```python
from build123d import *

# Parameters (mm, degrees)
F0_R     = 19.05
F0_R_2   = 6.35
F1_DEPTH = 38.1
F2_DEPTH = 12.7
F3_DEPTH = 6.35


with BuildPart() as f1:
    # F0 (on Top) → F1 (new body)
    with BuildSketch(Plane.XY):
        with BuildLine():
            ThreePointArc((-837.6395976841, 421.923872186), (-821.3424535269, 430.1577150999), (-814.7795976841, 447.1965530885))
            ThreePointArc((-814.7795976841, 447.1965530885), (-821.3424535269, 464.235391077), (-837.6395976841, 472.469233991))
            ThreePointArc((-837.6395976841, 472.469233991), (-865.5795976841, 447.1965530885), (-837.6395976841, 421.923872186))
        make_face()
        with Locations((-840.1795976841, 447.1965530885)):
            Circle(F0_R, mode=Mode.SUBTRACT)
        with BuildLine():
            ThreePointArc((-837.6395976841, 472.469233991), (-821.3424535269, 464.235391077), (-814.7795976841, 447.1965530885))
            ThreePointArc((-814.7795976841, 447.1965530885), (-821.3424535269, 430.1577150999), (-837.6395976841, 421.923872186))
            Line((-837.6395976841, 421.923872186), (-711.9095976841, 434.5602126372))
            ThreePointArc((-711.9095976841, 434.5602126372), (-725.8795976841, 447.1965530885), (-711.9095976841, 459.8328935397))
            Line((-711.9095976841, 459.8328935397), (-837.6395976841, 472.469233991))
        make_face()
        with BuildLine():
            ThreePointArc((-802.0795976841, 440.6483835481), (-808.6277672246, 447.1965530885), (-802.0795976841, 453.7447226289))
            Line((-802.0795976841, 453.7447226289), (-751.2795976841, 453.7447226289))
            ThreePointArc((-751.2795976841, 453.7447226289), (-744.7314281437, 447.1965530885), (-751.2795976841, 440.6483835481))
            Line((-751.2795976841, 440.6483835481), (-802.0795976841, 440.6483835481))
        make_face(mode=Mode.SUBTRACT)
        with BuildLine():
            ThreePointArc((-700.4795976841, 447.1965530885), (-703.7610256055, 455.7159720828), (-711.9095976841, 459.8328935397))
            ThreePointArc((-711.9095976841, 459.8328935397), (-725.8795976841, 447.1965530885), (-711.9095976841, 434.5602126372))
            ThreePointArc((-711.9095976841, 434.5602126372), (-703.7610256055, 438.6771340942), (-700.4795976841, 447.1965530885))
        make_face()
        with Locations((-713.1795976841, 447.1965530885)):
            Circle(F0_R_2, mode=Mode.SUBTRACT)
    extrude(amount=F1_DEPTH)

    # F0 (on Top) → F2 (cut)
    with BuildSketch(Plane.XY):
        with BuildLine():
            ThreePointArc((-837.6395976841, 472.469233991), (-821.3424535269, 464.235391077), (-814.7795976841, 447.1965530885))
            ThreePointArc((-814.7795976841, 447.1965530885), (-821.3424535269, 430.1577150999), (-837.6395976841, 421.923872186))
            Line((-837.6395976841, 421.923872186), (-711.9095976841, 434.5602126372))
            ThreePointArc((-711.9095976841, 434.5602126372), (-725.8795976841, 447.1965530885), (-711.9095976841, 459.8328935397))
            Line((-711.9095976841, 459.8328935397), (-837.6395976841, 472.469233991))
        make_face()
        with BuildLine():
            ThreePointArc((-802.0795976841, 440.6483835481), (-808.6277672246, 447.1965530885), (-802.0795976841, 453.7447226289))
            Line((-802.0795976841, 453.7447226289), (-751.2795976841, 453.7447226289))
            ThreePointArc((-751.2795976841, 453.7447226289), (-744.7314281437, 447.1965530885), (-751.2795976841, 440.6483835481))
            Line((-751.2795976841, 440.6483835481), (-802.0795976841, 440.6483835481))
        make_face(mode=Mode.SUBTRACT)
    extrude(amount=F2_DEPTH, mode=Mode.SUBTRACT)

    # F3 (cut): a face of the model
    f3_faces = [f1.faces().sort_by_distance(p)[0] for p in [
        (-714.4136766597, 459.4754838588, 0),
    ]]
    extrude(f3_faces, amount=-F3_DEPTH, mode=Mode.SUBTRACT)


solid = f1.part
```
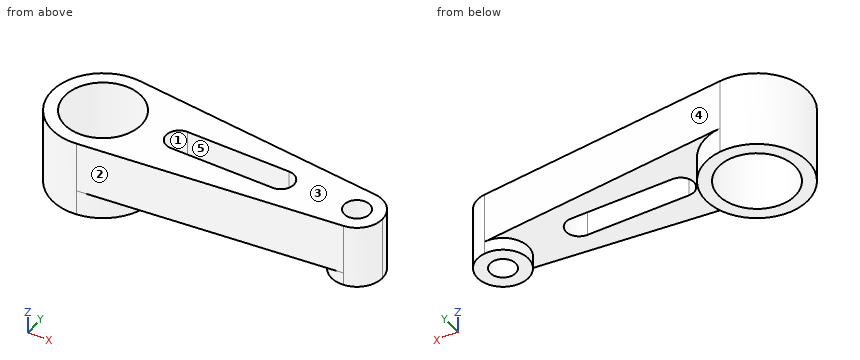
Verification items for the finished model (mm, model axes). Face numbers are marked on the shaded views. A direction names the side the tool comes from. Coordinates: 2 decimals unless noted, no trailing zeros. Write each loop counter-clockwise with the first axis right and the second up, starting at its lowest first coordinate (ties: lowest second). Pieces come first, ordered by that corner, then holes. Notation, with made-up numbers: (-1, 63) - (14, 63) arc R12 cw to (14, 81) - close; hole circle Ø4 at (21.25, 58.5). An arc over 180 degrees is marked (long way). Write item = value, one per line.
Q1. Mould release check, pull along Y, two halves, no side actions. Record for the marked faces 3, 4 and 5: released by +Y, released by -Y, zero draft, split by the parting line, or undercut.
Answer:
face_3 = zero draft
face_4 = released by +Y
face_5 = undercut
Q2. Access from +Z, -Z, +X, -X, +Y, -Y to the whole of each face (thin tool, end or side, straight path). Record for the marked faces 1 and 2.
Answer:
face_1 = +Z, -Z
face_2 = +Z, -Z, +X, -Y
Q3. Cross-section at B-B (x = -766). Enter the section's corners in (y, z), plus the area to 3 significant figures.
Answer:
outline = (429.12, 12.7) - (440.65, 12.7) - (440.65, 38.1) - (429.12, 38.1) - close; (453.74, 12.7) - (465.27, 12.7) - (465.27, 38.1) - (453.74, 38.1) - close
area = 585 mm²
Q4. Cross-section at C-C (y = 458). Enter the section's corners in (x, z), plus the area to 3 significant figures.
Answer:
outline = (-863.17, 0) - (-855.87, 0) - (-855.87, 38.1) - (-863.17, 38.1) - close; (-824.49, 0) - (-817.19, 0) - (-817.19, 12.7) - (-719.86, 12.7) - (-719.86, 6.35) - (-706.5, 6.35) - (-706.5, 38.1) - (-824.49, 38.1) - close
area = 3,450 mm²
Q5. Material ranges on L1, parallel to X at y = 445, z = 21.5; L2, parallel to X at y = 442, z = 15.5; L3, parallel to Z at x = -788.5, y = 435, recorded low to high. Write a range as from..to.
Answer:
L1 = -865.48..-859.1, -821.26..-808.25, -745.11..-719.14, -707.22..-700.67
L2 = -865.04..-858.51, -821.85..-806.06, -747.3..-716.83, -709.53..-701.59
L3 = 12.7..38.1
Q6. Cross-section at A-A (z = 8). Enter the section's corners in (x, y), plus the area to 3 significant figures.
Answer:
outline = circle Ø50.8 at (-840.18, 447.2); circle Ø25.4 at (-713.18, 447.2); hole circle Ø38.1 at (-840.18, 447.2); hole circle Ø12.7 at (-713.18, 447.2)
area = 1,270 mm²
Q7. Cross-section at D-D (z = 35). Enter the section's corners in (x, y), plus the area to 3 significant figures.
Answer:
outline = (-837.64, 421.92) - (-711.91, 434.56) arc R12.7 ccw to (-711.91, 459.83) - (-837.64, 472.47) arc R25.4 ccw (long way) to start; hole circle Ø38.1 at (-840.18, 447.2); hole (-802.08, 440.65) - (-751.28, 440.65) arc R6.55 ccw to (-751.28, 453.74) - (-802.08, 453.74) arc R6.55 ccw to start; hole circle Ø12.7 at (-713.18, 447.2)
area = 4,060 mm²
Q8. Go/stop test with flat-tipped pins: pin 1 Ø12 at (x, y) = (-768.5, 431.5) entering from -Z; pin 2 Ø3 at (x, z) = (-753.5, 19) entering from +Y; pin 3 Ø20.5 at (x, y) = (-712.5, 449.5) entering from -Z. Record where each tip stops, or that it passes through.
Answer:
pin_1 = 12.7
pin_2 = 464.16
pin_3 = 6.35
